Here's how the part is built. I have some questions about the finished solid (model axes, mm). A direction names the side the tool comes from. Coordinates: 2 decimals unless noted, no trailing zeros. Write each loop counter-clockwise with the first axis right and the second up, starting at its lowest first coordinate (ties: lowest second). Pieces come first, ordered by that corner, then holes. Notation, with made-up numbers: M 1.5,86.25 L 21.5,86.25 A15 ccw 21.5,91.25 Z; hole C 34,-14 d5. An arc over 180 degrees is marked long. Use a Markdown table: item, result.
Autodesk Inventor part; units mm, degrees
ref_plane "YZ Plane" through (0, 0, 0) normal (1, 0, 0) x (0, 1, 0)
ref_plane "XZ Plane" through (0, 0, 0) normal (0, 1, 0) x (-1, 0, 0)
ref_plane "XY Plane" through (0, 0, 0) normal (0, 0, 1) x (1, 0, 0)
sketch "Эскиз1" plane through (0, 0, 0) normal (0, 0, 1) x (1, 0, 0)
  circle A0 centre (0, 0) radius 12
  dimension "d0" = 24
extrude "Выдавливание1" add sketch "Эскиз1" along normal mid plane 37
sketch "Эскиз7" plane through (0, 0, 18.5) normal (0, 0, 1) x (1, 0, 0)
  circle A0 centre (0, 0) radius 13
  dimension "d27" = 26
extrude "Выдавливание7" add sketch "Эскиз7" along normal blind 4
mirror "Зеркальное отражение1" about plane through (0, 0, 0) normal (0, 0, 1) of "Выдавливание7"
sketch "Эскиз8" plane through (0, 0, 0) normal (1, 0, 0) x (0, 1, 0)
  circle A0 centre (0, 0) radius 12
  dimension "d30" = 24
extrude "Выдавливание8" add sketch "Эскиз8" against normal blind 14
sketch "Эскиз9" plane through (-14, 0, 0) normal (-1, 0, 0) x (0, 0, 1)
  circle A0 centre (0, 0) radius 13
  dimension "d33" = 26
extrude "Выдавливание9" add sketch "Эскиз9" along normal blind 4
sketch "Эскиз10" plane through (-18, 0, 0) normal (-1, 0, 0) x (0, 0, 1)
  circle A0 centre (0, 0) radius 10.4775
  dimension "d36" = 20.955
extrude "Выдавливание10" add sketch "Эскиз10" along normal blind 12
thread "Резьба1"
sketch "Эскиз11" plane through (0, 0, 22.5) normal (0, 0, 1) x (1, 0, 0)
  circle A0 centre (0, 0) radius 9.3155
  dimension "d41" = 18.631
extrude "Выдавливание11" cut sketch "Эскиз11" against normal through all
thread "Резьба2"
thread "Резьба3"
sketch "Эскиз12" plane through (-30, 0, 0) normal (-1, 0, 0) x (0, 0, 1)
  circle A0 centre (0, 0) radius 7.5
  dimension "d48" = 15
extrude "Выдавливание12" cut sketch "Эскиз12" against normal up to next
chamfer "Фаска5" distance 1.5 angle 45 1 edges at (-30, 0, -10.4775)
chamfer "Фаска6" distance 1.5 angle 45 1 edges at (-9.3155, 0, -22.5)
chamfer "Фаска7" distance 1.5 angle 45 1 edges at (-9.3155, 0, 22.5)
properties part number "Инж_граф_2"
1. Which directions (+Z, -Z, +X, -X, +Y, -Y) give clear straight access to the entire face, cutting with the end or side of a thin tool? Please do faces 4 (the face through (11.085, -4.596, 0.259)), 5 (the face through (-18, 6, -9)), 6 (the face through (-10.316, -7.91, -20.472)), 7 (the face through (-10.316, 7.91, 20.472)).
Answers follow:
| item | result |
|---|---|
| face 4 | none |
| face 5 | -X |
| face 6 | -Z |
| face 7 | +Z |
2. I need wall thicknesses on probe 1 along Y at (x, z) = (0, 12); probe 2 along X at (y, z) = (-1.5, -17); probe 3 along X at (y, z) = (-0.5, 6). Which ranges of each line are inside material? Lowest first, please.
Answers follow:
| item | result |
|---|---|
| probe 1 | y = -12 to -9.32, 9.32 to 12 |
| probe 2 | x = -11.91 to -9.19, 9.19 to 11.91 |
| probe 3 | x = 9.3 to 11.99 |
3. Suppose I cut it at A-A on z = 0. Write out the boundary of the cut face in (x, y).
Answers follow:
| item | result |
|---|---|
| outline | M -30,-8.98 L -28.5,-10.48 L -18,-10.48 L -18,-13 L -14,-13 L -14,-12 L 0,-12 A12 ccw 0,12 L -14,12 L -14,13 L -18,13 L -18,10.48 L -28.5,10.48 L -30,8.98 L -30,7.5 L -5.53,7.5 A9.32 cw long -5.53,-7.5 L -30,-7.5 Z |
4. Suppose I cut it at B-B on y = 0. State how many separate pieces and enclosed holes the cut face has, and give its area (3 significant figures).
Answers follow:
| item | result |
|---|---|
| separate pieces | 3 |
| enclosed holes | 0 |
| area | 344 mm2 |
5. Will these pins go through, and if not, where does the flat tip stop? pin 1 Ø5 at (x, z) = (-15.5, 3) entering from +Y; pin 2 Ø10 at (y, z) = (7, 8) entering from -X; pin 3 Ø13 at (x, y) = (-4, 1) entering from +Z; pin 4 Ø1.5 at (x, y) = (-25, -1) entering from +Z.
Answers follow:
| item | result |
|---|---|
| pin 1 | stops at y = 12.99 |
| pin 2 | stops at x = -30 |
| pin 3 | stops at z = 22.31 |
| pin 4 | stops at z = 10.47 |
6. We'd pull the mould along X, two halves only. Please class faces 1 (the face through (-30, -6, 5)), 2 (the face through (8.885, 2.798, 0.294)), 3 (the face through (-5, 10, 22.5)): +X half, -X half, draft (parallel to the pull), parting line (faces both ways), or undercut.
Answers follow:
| item | result |
|---|---|
| face 1 | -X half |
| face 2 | undercut |
| face 3 | draft |
7. Suppose I cut it at C-C on x = -20.5. Write out the boundary of the cut face in (y, z) (1 decimal), and give its area (3 significant figures).
Answers follow:
| item | result |
|---|---|
| outline | C 0,0 d21; hole C 0,0 d15 |
| area | 168 mm2 |
